Check sheet for the modelled part. Datum: model origin and axes. Units: mm. Give positions to 0.01 mm unless a question says otherwise; leave off trailing zeros. Write each loop counter-clockwise with the first axis right and the second up, starting at its lowest first coordinate (ties: lowest second). Pieces come first, ordered by that corner, then holes. Notation, with made-up numbers: M -14.5,1 L -10.5,1 A25 ccw -10.5,33 Z; hole C 44.5,28 d6. An arc over 180 degrees is marked long. Write item = value, one per line. Start each with the question number.
1) Cross-section at B-B, the plane x = -47.5. Record the cut outline in (y, z), plus the area to 3 significant figures.
2) Cross-section at A-A, the plane y = 19.5. Record the cut outline in (x, z).
3) Go/stop test with flat-tipped pins: pin 1 (0.9 mm diameter, centred on y = -81.5, z = 1, fed in from -X); pin 2 (0.9 mm diameter, centred on x = -89, z = 2, fed in from -Y). Record where each tip stops, or that it passes through.
4) Scan lines: line 1 along Y through (x, z) = (52, 0.95); line 2 along Y through (x, z) = (39, 0.2); line 3 along X through (y, z) = (15, 1.85). Record each from-to range of solid material in increasing order. Write a range as [from, to].
5) Cross-section at C-C, the plane z = 1.9. Give the number of separate pieces and of enclosed holes in the cut face, plus the area to 3 significant figures.
```python
from build123d import *

# Parameters (mm, degrees)
SKETCH1_R           = 50
BOSS_EXTRUDE1_DEPTH = 3
SKETCH2_R           = 1.6
CUT_EXTRUDE1_DEPTH  = 100.040395799
SKETCH3_R           = 1.6
CUT_EXTRUDE2_DEPTH  = 100.040395799
BOSS_EXTRUDE2_START = -3
SKETCH4_R           = 3.1
SKETCH4_W           = 140
SKETCH4_H           = 35
SKETCH4_R_2         = 3.2
BOSS_EXTRUDE2_DEPTH = 3
FILLET1_R           = 5
FILLET2_R           = 2


with BuildPart() as part:
    # Sketch1 → Boss-Extrude1 (new body)
    with BuildSketch(Plane.XY):
        with BuildLine():
            Line((-70, 0), (-70, -70))
            Line((-70, -70), (70, -70))
            Line((70, -70), (70, 0))
            ThreePointArc((70, 0), (0, 70), (-70, 0))
        make_face()
        Circle(SKETCH1_R, mode=Mode.SUBTRACT)
    extrude(amount=BOSS_EXTRUDE1_DEPTH)

    # Sketch2 → Cut-Extrude1 (cut, through all)
    with BuildSketch(Plane.XY.offset(3)):
        with Locations((0, 61)):
            Circle(SKETCH2_R)
        with Locations((52.827549631, 30.5)):
            Circle(SKETCH2_R)
        with Locations((52.827549631, -30.5)):
            Circle(SKETCH2_R)
        with Locations((0, -61)):
            Circle(SKETCH2_R)
        with Locations((-52.827549631, -30.5)):
            Circle(SKETCH2_R)
        with Locations((-52.827549631, 30.5)):
            Circle(SKETCH2_R)
    extrude(amount=-CUT_EXTRUDE1_DEPTH, mode=Mode.SUBTRACT)

    # Sketch3 → Cut-Extrude2 (cut, through all)
    with BuildSketch(Plane.XY.offset(3)):
        with Locations((14.235047481, 53.125920446)):
            Circle(SKETCH3_R)
        with Locations((38.890872965, 38.890872965)):
            Circle(SKETCH3_R)
        with Locations((53.125920446, 14.235047481)):
            Circle(SKETCH3_R)
        with Locations((53.125920446, -14.235047481)):
            Circle(SKETCH3_R)
        with Locations((38.890872965, -38.890872965)):
            Circle(SKETCH3_R)
        with Locations((14.235047481, -53.125920446)):
            Circle(SKETCH3_R)
        with Locations((-14.235047481, -53.125920446)):
            Circle(SKETCH3_R)
        with Locations((-38.890872965, -38.890872965)):
            Circle(SKETCH3_R)
        with Locations((-53.125920446, -14.235047481)):
            Circle(SKETCH3_R)
        with Locations((-53.125920446, 14.235047481)):
            Circle(SKETCH3_R)
        with Locations((-38.890872965, 38.890872965)):
            Circle(SKETCH3_R)
        with Locations((-14.235047481, 53.125920446)):
            Circle(SKETCH3_R)
    extrude(amount=-CUT_EXTRUDE2_DEPTH, mode=Mode.SUBTRACT)

    # Sketch4 → Boss-Extrude2 (add)
    # profile 1 of 3: a face of its own
    with BuildSketch(Plane.XY.offset(3).offset(BOSS_EXTRUDE2_START)):
        with BuildLine():
            ThreePointArc((-70, 0), (-69.592305666, 7.543937436), (-68.373971656, 15))
            Line((-68.373971656, 15), (-105, -48.438141971))
            Line((-105, -48.438141971), (-105, -70))
            Line((-105, -70), (-70, -70))
            Line((-70, -70), (-70, 0))
        make_face()
        with Locations((-90, -55)):
            Circle(SKETCH4_R, mode=Mode.SUBTRACT)
    # profile 2 of 3: a face of its own
    with BuildSketch(Plane.XY.offset(3).offset(BOSS_EXTRUDE2_START)):
        with BuildLine():
            Line((105, -48.438141971), (68.373971656, 15))
            ThreePointArc((68.373971656, 15), (69.592305666, 7.543937436), (70, 0))
            Line((70, 0), (70, -70))
            Line((70, -70), (105, -70))
            Line((105, -70), (105, -48.438141971))
        make_face()
        with Locations((90, -55)):
            Circle(SKETCH4_R, mode=Mode.SUBTRACT)
    # profile 3 of 3: a face of its own
    with BuildSketch(Plane.XY.offset(3).offset(BOSS_EXTRUDE2_START)):
        with Locations((0, -87.5)):
            Rectangle(SKETCH4_W, SKETCH4_H)
        with Locations((-40, -90)):
            Circle(SKETCH4_R_2, mode=Mode.SUBTRACT)
        with Locations((40, -90)):
            Circle(SKETCH4_R_2, mode=Mode.SUBTRACT)
    extrude(amount=BOSS_EXTRUDE2_DEPTH)

    # Fillet1
    fillet1_edges = [part.edges().sort_by_distance(p)[0] for p in [
        (-105, -70, 1.5),
        (-105, -48.438141971, 1.5),
        (-68.373971656, 15, 1.5),
        (68.373971656, 15, 1.5),
        (105, -48.438141971, 1.5),
        (105, -70, 1.5),
        (-70, -105, 1.5),
        (70, -105, 1.5),
    ]]
    fillet(fillet1_edges, radius=FILLET1_R)

    # Fillet2
    fillet2_edges = [part.edges().sort_by_distance(p)[0] for p in [
        (-70, -70, 1.5),
        (70, -70, 1.5),
    ]]
    fillet(fillet2_edges, radius=FILLET2_R)


solid = part.part
```
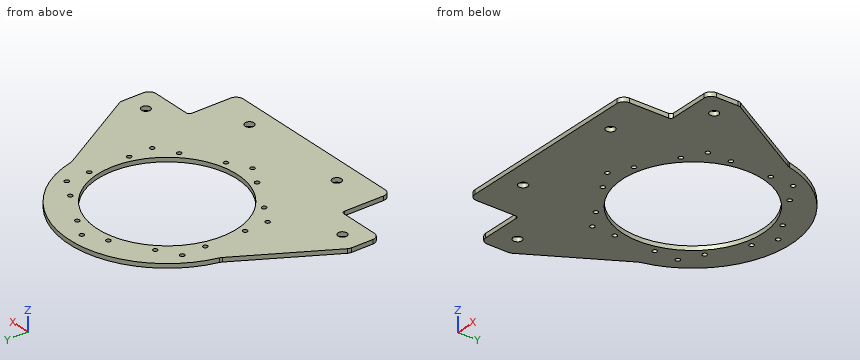
Reply:
q1.outline = M -105,0 L -15.61,0 L -15.61,3 L -105,3 Z; M 15.61,0 L 51.42,0 L 51.42,3 L 15.61,3 Z
q1.area = 376 mm2
q2.outline = M -67.23,0 L -46.04,0 L -46.04,3 L -67.23,3 Z; M 46.04,0 L 67.23,0 L 67.23,3 L 46.04,3 Z
q3.pin_1 = -70
q3.pin_2 = -70
q4.line_1 = [-105, -31.87], [-29.13, -15.37], [-13.1, 13.1], [15.37, 29.13], [31.87, 46.86]
q4.line_2 = [-105, -93.04], [-86.96, -40.49], [-37.29, -31.29], [31.29, 37.29], [40.49, 58.13]
q4.line_3 = [-68.44, -54.53], [-51.72, -47.7], [47.7, 51.72], [54.53, 68.44]
q5.separate_pieces = 1
q5.enclosed_holes = 23
q5.area = 17,900 mm2
